Design review of the part built by this model. Coordinates are the model's own, in mm. Face numbers are marked on the shaded views. A direction names the side the tool comes from. Coordinates: 2 decimals unless noted, no trailing zeros. Write each loop counter-clockwise with the first axis right and the second up, starting at its lowest first coordinate (ties: lowest second). Pieces come first, ordered by that corner, then holes.
Q1. Add section D-D, the plane y = 3.5. Give the boundary of the cut face in (x, z).
Q2. Add section A-A, the plane y = 9.06. Give the boundary of the cut face in (x, z), plus the area to 3 significant figures.
Q3. Add section C-C, the plane z = 2.35. Give the boundary of the cut face in (x, y), plus the area to 3 significant figures.
Q4. Clearance check with flat-ended pins moving along their axes: pin 1 Ø1.5 at (y, z) = (-7, 2.5) entering from -X; pin 2 Ø3 at (x, y) = (15, 9.06) entering from -Z. State where each tip first meets the part, or that it passes through.
Q5. To check wall thickness, follow probe 1 along Y at (x, z) = (-15, 3.2); probe 2 along Y at (x, z) = (22, 1.5); probe 3 along X at (y, z) = (9.5, 2.15). State the ranges of each line that lie inside material, in increasing order.
Q6. Machinability: for the marked faces 4, 5 and 6, which of the approach directions +Z, -Z, +X, -X, +Y, -Y give a long, thin tool a straight path to every point of the face, cutting with its end or side? Answer none if there is none.
Q7. The part is to be moulded in two halves that separate along Y. For the marked faces 1, 2 and 3, say which applies: +Y half, -Y half, draft (parallel to the pull), parting line (faces both ways), or undercut.
Q8. Add section B-B, the plane x = -15. Give the boundary of the cut face in (y, z), plus the area to 3 significant figures.
Autodesk Inventor part; units mm, degrees
ref_plane "YZ Plane" through (0, 0, 0) normal (1, 0, 0) x (0, 1, 0)
ref_plane "XZ Plane" through (0, 0, 0) normal (0, 1, 0) x (-1, 0, 0)
ref_plane "XY Plane" through (0, 0, 0) normal (0, 0, 1) x (1, 0, 0)
sketch "Sketch1" plane through (0, 0, 0) normal (0, 0, 1) x (1, 0, 0)
  line L0 (20.01, -20) -> (-20.01, -20)
  line L1 (-20.01, -20) -> (-20.01, 20)
  line L2 (-20.01, 20) -> (20.01, 20)
  line L3 (20.01, 20) -> (20.01, -20)
  line L4 (20.01, -20) -> (-20.01, 20) construction
  line L5 (-20.01, -20) -> (20.01, 20) construction
  line L6 (-20.01, 20) -> (-25.11, 20)
  line L7 (-25.11, 20) -> (-25.11, -20)
  line L8 (-25.11, -20) -> (-20.01, -20)
  line L9 (-20.01, -20) -> (-20.01, 20)
  line L10 (20.01, 20) -> (25.11, 20)
  line L11 (25.11, 20) -> (25.11, -20)
  line L12 (25.11, -20) -> (20.01, -20)
  line L13 (20.01, -20) -> (20.01, 20)
  point P0 (0, 0)
  point P1 (20.01, -20)
  dimension "d0" = 40.02
  dimension "d1" = 40
  dimension "d2" = 5.1
  dimension "d3" = 5.1
extrude "Extrusion1" add sketch "Sketch1" along normal blind 5.1 contours L0 L1 L2 L3
sketch "Sketch3" plane through (0, 0, 0) normal (0, 0, -1) x (-1, 0, 0)
  circle A0 centre (15, -15) radius 2
  circle A1 centre (-15, -15) radius 2
  circle A2 centre (15, 9.06) radius 2
  circle A3 centre (-15, 9.06) radius 2
  point P0 (0, 0)
  dimension "d8" = 4
  dimension "d9" = 4
  dimension "d10" = 4
  dimension "d11" = 4
  dimension "d12" = 15
  dimension "d14" = 15
  dimension "d16" = 15
  dimension "d17" = 15
  dimension "d18" = 15
  dimension "d19" = 15
  dimension "d30" = 24.06
  dimension "d31" = 24.06
extrude "Extrusion3" cut sketch "Sketch3" against normal blind 10
thread "Thread1"
thread "Thread2"
thread "Thread3"
thread "Thread4"
sketch "Sketch4" plane through (0, 0, 0) normal (0, 0, -1) x (-1, 0, 0)
  line L0 (20.01, 20) -> (20.01, -20)
  line L1 (20.01, -10) -> (14.91, -10)
  line L2 (14.91, -10) -> (14.91, -4.5)
  line L3 (14.91, -4.5) -> (20.01, -4.5)
  line L4 (20.01, -4.5) -> (20.01, -10)
  line L5 (20.01, -20) -> (-20.01, -20)
  line L6 (20.01, 0.6) -> (14.91, 0.6)
  line L7 (14.91, 0.6) -> (14.91, 6.1)
  line L8 (14.91, 6.1) -> (20.01, 6.1)
  line L9 (20.01, 6.1) -> (20.01, 0.6)
  line L10 (-20.01, 20) -> (20.01, 20)
  line L11 (0, 0) -> (0, -7.4) construction
  line L12 (-20.01, -10) -> (-14.91, -10)
  line L13 (-14.91, -10) -> (-14.91, -4.5)
  line L14 (-14.91, -4.5) -> (-20.01, -4.5)
  line L15 (-20.01, -4.5) -> (-20.01, -10)
  line L16 (-20.01, 0.6) -> (-14.91, 0.6)
  line L17 (-14.91, 0.6) -> (-14.91, 6.1)
  line L18 (-14.91, 6.1) -> (-20.01, 6.1)
  line L19 (-20.01, 6.1) -> (-20.01, 0.6)
  dimension "d32" = 5.1
  dimension "d33" = 5.5
  dimension "d34" = 10
  dimension "d35" = 5.1
  dimension "d36" = 5.5
  dimension "d37" = 13.9
extrude "Extrusion4" cut sketch "Sketch4" against normal blind 10
sketch "Sketch5" plane through (-20.01, -20, 0) normal (-1, 0, 0) x (0, 0, 1)
  line L0 (5.1, 10) -> (0, 10)
  line L1 (0, 10) -> (0, 0)
  line L2 (0, 0) -> (5.1, 0)
  line L3 (5.1, 10) -> (5.1, 0)
  line L4 (5.1, 20.6) -> (0, 20.6)
  line L5 (0, 20.6) -> (0, 15.5)
  line L6 (0, 15.5) -> (5.1, 15.5)
  line L7 (5.1, 20.6) -> (5.1, 15.5)
  line L8 (0, 26.1) -> (5.1, 26.1)
  line L9 (5.1, 40) -> (5.1, 26.1)
  line L10 (0, 40) -> (5.1, 40)
  line L11 (0, 40) -> (0, 26.1)
  point P0 (0, 20)
extrude "Extrusion5" add sketch "Sketch5" along normal blind 5.1
sketch "Sketch6" plane through (20.01, -20, 5.1) normal (1, 0, 0) x (0, 0, -1)
  line L0 (5.1, 10) -> (0, 10)
  line L1 (0, 0) -> (0, 10)
  line L2 (5.1, 0) -> (0, 0)
  line L3 (5.1, 0) -> (5.1, 10)
  line L4 (0, 15.5) -> (5.1, 15.5)
  line L5 (5.1, 15.5) -> (5.1, 20.6)
  line L6 (5.1, 20.6) -> (0, 20.6)
  line L7 (0, 15.5) -> (0, 20.6)
  line L8 (5.1, 31.06) -> (0, 31.06)
  line L9 (0, 26.1) -> (5.1, 26.1)
  line L10 (5.1, 26.1) -> (5.1, 40)
  line L11 (5.1, 40) -> (0, 40)
  line L12 (0, 26.1) -> (0, 40)
  point P0 (5.1, 20)
extrude "Extrusion6" add sketch "Sketch6" along normal blind 5.1
sketch "Sketch7" plane through (0, 0, 0) normal (0, 0, -1) x (-1, 0, 0)
  line L0 (14.91, -10) -> (14.91, -4.5)
  line L1 (14.91, -10) -> (25.11, -10)
  line L2 (14.91, -4.5) -> (20.01, -4.5)
  line L3 (20.01, -4.5) -> (20.01, -10)
  line L4 (20.01, -10) -> (14.91, -10)
  line L5 (14.91, -10) -> (14.91, -4.5)
  line L6 (14.91, 0.6) -> (14.91, 6.1)
  line L7 (14.91, 6.1) -> (25.11, 6.1)
  line L8 (14.91, 0.6) -> (20.01, 0.6)
  line L9 (20.01, 0.6) -> (20.01, 6.1)
  line L10 (20.01, 6.1) -> (14.91, 6.1)
  line L11 (14.91, 6.1) -> (14.91, 0.6)
  line L12 (-14.91, -10) -> (-25.11, -10)
  line L13 (-14.91, -4.5) -> (-25.11, -4.5)
  line L14 (-14.91, -10) -> (-20.01, -10)
  line L15 (-20.01, -10) -> (-20.01, -4.5)
  line L16 (-20.01, -4.5) -> (-14.91, -4.5)
  line L17 (-14.91, -4.5) -> (-14.91, -10)
  line L18 (-14.91, 6.1) -> (-14.91, 0.6)
  line L19 (-14.91, 0.6) -> (-25.11, 0.6)
  line L20 (-14.91, 6.1) -> (-20.01, 6.1)
  line L21 (-20.01, 6.1) -> (-20.01, 0.6)
  line L22 (-20.01, 0.6) -> (-14.91, 0.6)
  line L23 (-14.91, 0.6) -> (-14.91, 6.1)
  point P0 (0, 0)
  dimension "d44" = 5.1
  dimension "d45" = 5.1
extrude "Extrusion7" add sketch "Sketch7" against normal blind 5.1
properties part number "caster wheel mounter" material "Polycarbonate, Clear"
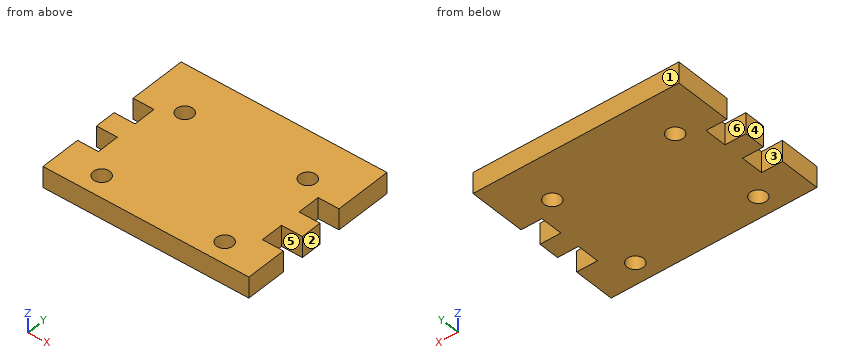
Here are the results:
1. outline: (-20.01, 0) - (20.01, 0) - (20.01, 5.1) - (-20.01, 5.1) - close
2. outline: (-25.11, 0) - (-17, 0) - (-17, 5.1) - (-25.11, 5.1) - close; (-13, 0) - (13, 0) - (13, 5.1) - (-13, 5.1) - close; (17, 0) - (25.11, 0) - (25.11, 5.1) - (17, 5.1) - close
2. area: 215 mm2
3. outline: (-25.11, -20) - (25.11, -20) - (25.11, -10) - (20.01, -10) - (20.01, -4.5) - (25.11, -4.5) - (25.11, 0.6) - (20.01, 0.6) - (20.01, 6.1) - (25.11, 6.1) - (25.11, 20) - (-25.11, 20) - (-25.11, 6.1) - (-20.01, 6.1) - (-20.01, 0.6) - (-25.11, 0.6) - (-25.11, -4.5) - (-20.01, -4.5) - (-20.01, -10) - (-25.11, -10) - close; hole circle Ø4 at (-15, -15); hole circle Ø4 at (-15, 9.06); hole circle Ø4 at (15, -15); hole circle Ø4 at (15, 9.06)
3. area: 1,850 mm2
4. pin 1: stops at x = -20.01
4. pin 2: passes through
5. probe 1: y = -20 to -17, -13 to 7.06, 11.06 to 20
5. probe 2: y = -20 to -10, -4.5 to 0.6, 6.1 to 20
5. probe 3: x = -25.11 to -16.95, -13.05 to 13.05, 16.95 to 25.11
6. face 4: +Z, -Z, -X, +Y, -Y
6. face 5: +Z, -Z, +X
6. face 6: +Z, -Z, -X
7. face 1: +Y half
7. face 2: draft
7. face 3: undercut
8. outline: (-20, 0) - (-17, 0) - (-17, 5.1) - (-20, 5.1) - close; (-13, 0) - (7.06, 0) - (7.06, 5.1) - (-13, 5.1) - close; (11.06, 0) - (20, 0) - (20, 5.1) - (11.06, 5.1) - close
8. area: 163 mm2
